The listing builds one solid part. Answer for the finished solid, in the listing's coordinates (mm). Face numbers are marked on the shaded views. A direction names the side the tool comes from. Give positions to 0.01 mm unless a question says otherwise; leave off trailing zeros. Order: outer loops, then holes, each group sorted by start corner. A loop starts at its lowest first (then second) coordinate and runs counter-clockwise, first axis right, second up.
```python
from build123d import *

# Parameters (mm, degrees)
SKETCH1_W           = 6.35
SKETCH1_H           = 6.35
BOSS_EXTRUDE1_DEPTH = 4.7625
FILLET1_R           = 3.175


with BuildPart() as part:
    # Sketch1 → Boss-Extrude1 (new body, symmetric)
    with BuildSketch(Plane(origin=(0, 0, 0), x_dir=(1, 0, 0), z_dir=(0, 1, 0))):
        with BuildLine():
            Line((40.80332125, -0.381), (60.325, -0.381))
            Line((60.325, -0.381), (60.325, -3.96875))
            Line((60.325, -3.96875), (47.086170591, -3.96875))
            ThreePointArc((47.086170591, -3.96875), (2.8406806, -44.365205708), (-45.900442536, -9.525))
            Line((-45.900442536, -9.525), (-60.325, -9.525))
            Line((-60.325, -9.525), (-60.325, 9.525))
            Line((-60.325, 9.525), (-45.900442536, 9.525))
            ThreePointArc((-45.900442536, 9.525), (2.8406806, 44.365205708), (47.086170591, 3.96875))
            Line((47.086170591, 3.96875), (60.325, 3.96875))
            Line((60.325, 3.96875), (60.325, 0.381))
            Line((60.325, 0.381), (40.80332125, 0.381))
            ThreePointArc((40.80332125, 0.381), (-40.8051, 0), (40.80332125, -0.381))
        make_face()
        with Locations((-50.8, 0)):
            Rectangle(SKETCH1_W, SKETCH1_H, mode=Mode.SUBTRACT)
    extrude(amount=BOSS_EXTRUDE1_DEPTH, both=True)

    # Fillet1
    fillet1_edges = [part.edges().sort_by_distance(p)[0] for p in [
        (-45.900442536, 0, 9.525),
        (-60.325, 0, 9.525),
        (-60.325, 0, -9.525),
        (-45.900442536, 0, -9.525),
        (47.086170591, 0, -3.96875),
        (47.086170591, 0, 3.96875),
    ]]
    fillet(fillet1_edges, radius=FILLET1_R)


solid = part.part
```
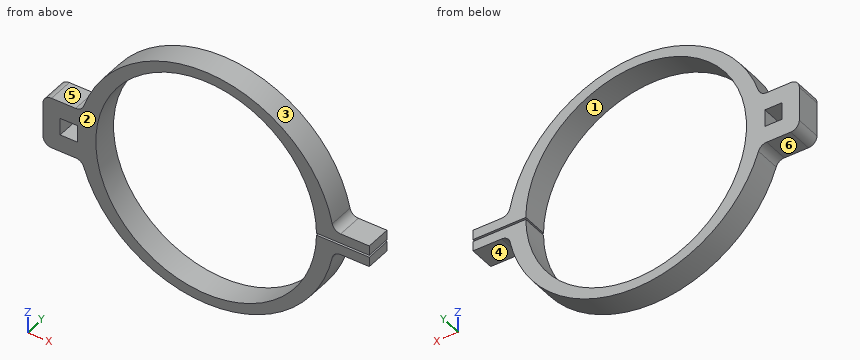
1) Find section B-B (z = 13). Write down the section's boundary in (x, y).
Geometry says:
outline: (-44.79, -4.76) - (-38.68, -4.76) - (-38.68, 4.76) - (-44.79, 4.76) - close; (38.68, -4.76) - (44.79, -4.76) - (44.79, 4.76) - (38.68, 4.76) - close
2) Find section C-C (y = -1). Write down the section's boundary in (x, z) (3 decimals), then the cut area to 3 significant figures.
Geometry says:
outline: (-60.325, -6.35) arc R3.175 ccw to (-57.15, -9.525) - (-48.256, -9.525) arc R3.175 cw to (-45.24, -11.708) arc R47.625 ccw to (46.632, -6.499) arc R3.175 cw to (49.741, -3.969) - (60.325, -3.969) - (60.325, -0.381) - (40.803, -0.381) arc R40.805 cw (long way) to (40.803, 0.381) - (60.325, 0.381) - (60.325, 3.969) - (49.741, 3.969) arc R3.175 cw to (46.632, 6.499) arc R47.625 ccw to (-45.24, 11.708) arc R3.175 cw to (-48.256, 9.525) - (-57.15, 9.525) arc R3.175 ccw to (-60.325, 6.35) - close; hole (-53.975, -3.175) - (-47.625, -3.175) - (-47.625, 3.175) - (-53.975, 3.175) - close
area: 1,590 mm2
3) For a pull along Z with two mould halves and no side action, classify the marked faces 1, 2 and 3 as +Z half, -Z half, draft (parallel to the pull), parting line (faces both ways), or undercut.
Geometry says:
face 1: undercut
face 2: draft
face 3: +Z half
4) A tool of negligible diameter and unlimited length cuts with its end or side. For the marked faces 4, 5 and 6, from which of +Z, -Z, +X, -X, +Y, -Y can it reach the whole face along a straight path? Write none if from no direction.
Geometry says:
face 4: -Z, +X, +Y, -Y
face 5: +Z, -X, +Y, -Y
face 6: -Z, -X, +Y, -Y
5) Given P1, Ø5, axis at x = -51, y = -0.5, coming from the -Z side (3 decimals); P2, Ø2.5, axis at x = -53.5, y = 1.5, coming from the +Z side (3 decimals); P3, Ø1.5, axis at x = 31, y = -2, coming from the +Z side, each flat-ended and moving along its own axis, determine where each tip first touches the part or whether it passes through.
Geometry says:
P1: stops at z = -9.525
P2: stops at z = 9.525
P3: stops at z = 33.61
6) Find section A-A (x = 0). Write down the section's boundary in (y, z), then the cut area to 3 significant figures.
Geometry says:
outline: (-4.76, -44.45) - (4.76, -44.45) - (4.76, -40.81) - (-4.76, -40.81) - close; (-4.76, 40.81) - (4.76, 40.81) - (4.76, 44.45) - (-4.76, 44.45) - close
area: 69.4 mm2
7) Straight lines are drawn through the part: probe 1 along X at (y, z) = (-2.5, 0) (3 decimals); probe 2 along Z at (x, y) = (0, -0.75); probe 3 along Z at (x, y) = (-49, -2.5) (3 decimals). For each, find the intervals that lie inside material, in ascending order.
Geometry says:
probe 1: x = -60.325 to -53.975, -47.625 to -40.805
probe 2: z = -44.45 to -40.81, 40.81 to 44.45
probe 3: z = -9.525 to -3.175, 3.175 to 9.525
